Drawing for the job (mm, zero at the part's lowest x, y, z). Coordinates: 2 decimals unless noted, no trailing zeros. Loops run counter-clockwise (first coordinate to the right, second up) from the corner with the lowest first, then second, coordinate; pieces in that order, holes last. Notation, with made-up numbers: (29, 60) -> (49, 60) arc R7 cw to (49, 70) -> close; hole circle Ø5 at (32.5, 53.25). An arc over 180 degrees is marked (long way). Write item = value, one per line. Start each with the question number.
(1) Flat gauge pins, fed straight in: P1, Ø3, axis at x = 10, y = 13, coming from the -Z side; P2, Ø4, axis at x = 6.35, y = 7.33, coming from the -Z side; P3, Ø3, axis at x = 9.5, z = 51.5, coming from the +Y side; P4, Ø4.5, axis at x = 6.35, y = 7.33, coming from the +Z side. Where does each tip first touch, or does it go through?
(2) Band-saw the part on C-C (x = 2). Write the cut outline in (y, z) (1 decimal).
(3) Drill centre lines: line 1 (Y direction, x = 6.35, z = 85.5) (1 decimal); line 2 (Y direction, x = 7, z = 77.5) (1 decimal); line 3 (X direction, y = 6.5, z = 17). Where is each one in solid material? Low to high. Write a range as from..to.
(4) Band-saw the part on D-D (y = 1). Write the cut outline in (x, z) (1 decimal).
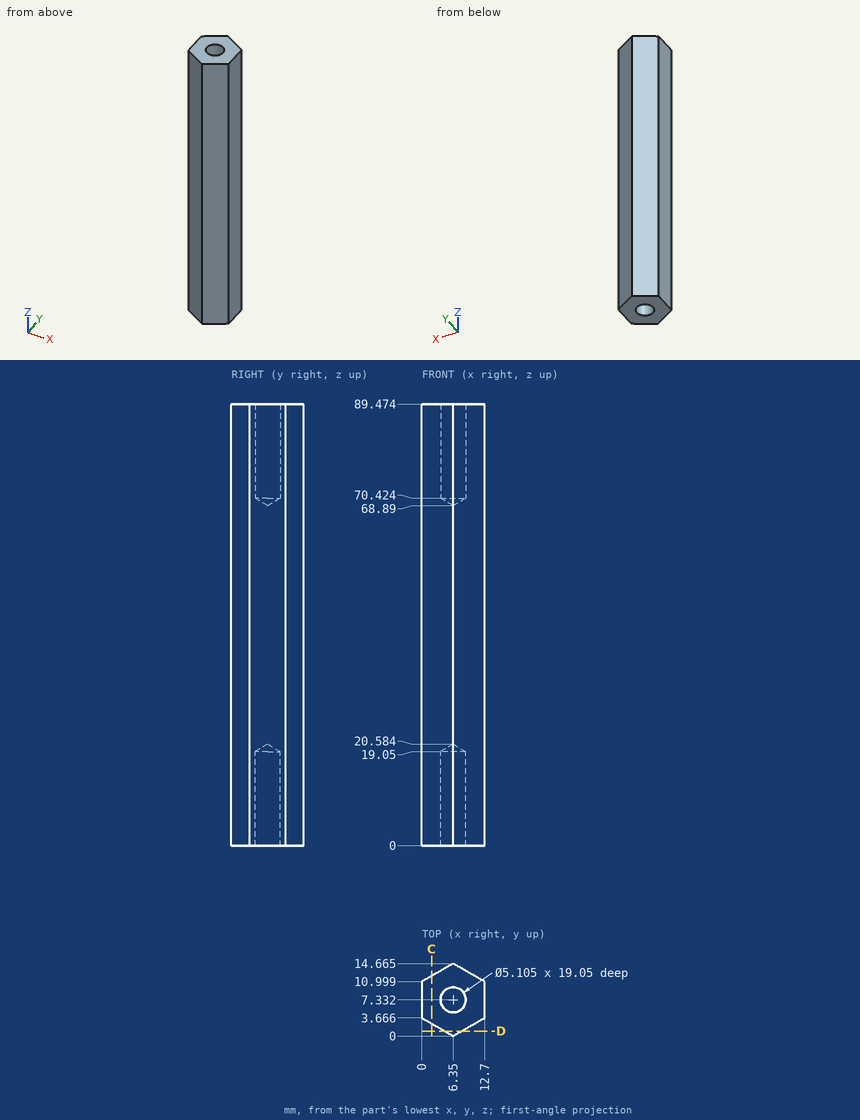
Findings below:
q1.P1 = 0
q1.P2 = 19.38
q1.P3 = 13.71
q1.P4 = 70.24
q2.outline = (2.5, 0) -> (12.2, 0) -> (12.2, 89.5) -> (2.5, 89.5) -> close
q3.line_1 = 0..4.8, 9.9..14.7
q3.line_2 = 0.4..4.9, 9.8..14.3
q3.line_3 = 0..3.94, 8.76..12.7
q4.outline = (4.6, 0) -> (8.1, 0) -> (8.1, 89.5) -> (4.6, 89.5) -> close
